Read the model definition and answer for the solid it produces. Units are mm, in the model's axes. Face numbers are marked on the shaded views. A direction names the side the tool comes from. Round coordinates to 2 decimals unless told otherwise and drop trailing zeros. Order: outer loops, then holes, each group sorted by start corner. A loop starts at its lowest first (then second) coordinate and runs counter-clockwise, first axis right, second up. Notation, with made-up numbers: (67, 37) - (81, 37) arc R26 ccw to (81, 53) - close; hole circle Ø11 at (-14, -2). An arc over 180 degrees is marked (long way). Put each result on its own line as item: value. Start each with the question number.
Q1. Section A-A on x = 103 is taken. Give the vertices of the cut face in (y, z), then the cut area to 3 significant figures.
Q2. Find the intervals of material crossed by line 1 along X through (y, z) = (216, -268); line 2 along X through (y, z) = (22, -107.5); line 3 along Z through (x, y) = (-50.5, 80.5), in increasing order. Write a range as from..to.
Q3. Which of the six approach directions +Z, -Z, +X, -X, +Y, -Y give full straight-line access (tool end or side, diameter ignored) to the marked faces 1, 2 and 3?
Q4. Section B-B on z = -290 is taken. Give the vertices of the cut face in (x, y), then the cut area to 3 significant figures.
Q5. Each of these flat-tipped pins is pushed along its axis until it touches: pin 1 Ø5.5 at (y, z) = (24.5, -353) entering from +X; pin 2 Ø5 at (x, y) = (9, -41) entering from +Z; pin 3 Ø10.5 at (x, z) = (3.5, -203.5) entering from +Y. Where does it stop, or does it pass through?
Q6. For a pull along Y with two mould halves and no side action, classify the marked faces 4, 5, 6 and 7 as pulls with the +Y half, pulls with the -Y half, needs draft (parallel to the pull), parting line crosses it, or undercut.
from build123d import *

# Parameters (mm, degrees)
SKETCH3_R           = 8.765690973
SKETCH3_R_2         = 7.546329472
BOSS_EXTRUDE1_DEPTH = 33.02
SKETCH3_3_R         = 8.765690973
SKETCH3_3_R_2       = 4.747089374
BOSS_EXTRUDE2_DEPTH = 69.85
BOSS_EXTRUDE3_START = 58.42
SKETCH3_4_R         = 8.765690973
BOSS_EXTRUDE3_DEPTH = 25.4
BOSS_EXTRUDE4_START = 147.32
SKETCH3_5_R         = 37.933984784
BOSS_EXTRUDE4_DEPTH = 88.9
BOSS_EXTRUDE5_START = -33.02
SKETCH3_6_R         = 8.765690973
BOSS_EXTRUDE5_DEPTH = 36.83
SKETCH4_R           = 29.883477217
SKETCH4_R_2         = 43.238390789
BOSS_EXTRUDE6_DEPTH = 63.5
SKETCH5_R           = 12.7
BOSS_EXTRUDE7_DEPTH = 76.2


with BuildPart() as part:
    # Sketch3 → Boss-Extrude1 (new, symmetric)
    with BuildSketch(Plane(origin=(0, 0, 0), x_dir=(0, 0, -1), z_dir=(1, 0, 0))):
        with BuildLine():
            Line((26.855598623, 34.04153134), (4.47810231, 12.180709193))
            ThreePointArc((4.47810231, 12.180709193), (-0.623125102, -0.971268934), (5.942795811, -13.456689726))
            Line((5.942795811, -13.456689726), (66.019432644, -60.042158643))
            ThreePointArc((66.019432644, -60.042158643), (76.890934177, -67.24165573), (88.712417559, -72.743912948))
            Line((88.712417559, -72.743912948), (111.45096516, -102.748262935))
            Line((111.45096516, -102.748262935), (144.477083252, -102.748262935))
            Line((144.477083252, -102.748262935), (169.002654574, -78.222691613))
            Line((169.002654574, -78.222691613), (195.607463956, -67.881296304))
            Line((195.607463956, -67.881296304), (230.151439421, -67.881296304))
            Line((230.151439421, -67.881296304), (255.413307952, -58.06190745))
            Line((255.413307952, -58.06190745), (278.88283078, -45.976265865))
            ThreePointArc((278.88283078, -45.976265865), (294.32962444, -40.865539072), (306.21453812, -29.753753007))
            Line((306.21453812, -29.753753007), (343.20837466, -16.328313428))
            Line((343.20837466, -16.328313428), (371.754392863, 12.180709193))
            Line((371.754392863, 12.180709193), (374.485546232, 37.116975937))
            Line((374.485546232, 37.116975937), (357.663762198, 55.324665065))
            Line((357.663762198, 55.324665065), (334.531136252, 76.90543329))
            Line((334.531136252, 76.90543329), (344.934785387, 122.683933603))
            Line((344.934785387, 122.683933603), (364.263564291, 181.676846378))
            Line((364.263564291, 181.676846378), (364.263564291, 198.452389962))
            Line((364.263564291, 198.452389962), (357.663762198, 223.699422208))
            Line((357.663762198, 223.699422208), (344.934785387, 227.677887566))
            Line((344.934785387, 227.677887566), (344.934785387, 233.598698071))
            Line((344.934785387, 233.598698071), (249.548191735, 247.947506817))
            Line((249.548191735, 247.947506817), (244.248903474, 242.648218557))
            Line((244.248903474, 242.648218557), (232.751756038, 242.648218557))
            Line((232.751756038, 242.648218557), (227.094867147, 224.549177586))
            Line((227.094867147, 224.549177586), (219.151380314, 218.377908492))
            Line((219.151380314, 218.377908492), (211.768889899, 192.707825641))
            Line((211.768889899, 192.707825641), (198.41781103, 192.707825641))
            Line((198.41781103, 192.707825641), (186.570468216, 151.512747216))
            Line((186.570468216, 151.512747216), (220.727605993, 147.448698974))
            Line((220.727605993, 147.448698974), (210.286236359, 90.83239142))
            Line((210.286236359, 90.83239142), (139.553233817, 50.621163948))
            Line((139.553233817, 50.621163948), (99.972286673, 57.295598172))
            Line((99.972286673, 57.295598172), (49.830851017, 45.21297855))
            Line((49.830851017, 45.21297855), (26.855598623, 34.04153134))
        make_face()
        with Locations((354.042271494, 27.57532186)):
            Circle(SKETCH3_R, mode=Mode.SUBTRACT)
        with Locations((16.377571024, 0)):
            Circle(SKETCH3_R_2, mode=Mode.SUBTRACT)
    extrude(amount=BOSS_EXTRUDE1_DEPTH, both=True)



with BuildPart() as body_2:
    # Sketch3<3> → Boss-Extrude2 (new, symmetric)
    with BuildSketch(Plane(origin=(0, 0, 0), x_dir=(0, 0, -1), z_dir=(1, 0, 0))):
        with Locations((354.042271494, 27.57532186)):
            Circle(SKETCH3_3_R)
        with Locations((354.042271494, 27.57532186)):
            Circle(SKETCH3_3_R_2, mode=Mode.SUBTRACT)
    extrude(amount=BOSS_EXTRUDE2_DEPTH, both=True)


with BuildPart() as part_1:
    add(part.part)

    add(body_2.part)  # Boss-Extrude3 merges body 2
    # Sketch3<4> → Boss-Extrude3 (add)
    with BuildSketch(Plane(origin=(0, 0, 0), x_dir=(0, 0, -1), z_dir=(1, 0, 0)).offset(BOSS_EXTRUDE3_START)):
        with BuildLine():
            ThreePointArc((32.215659867, 6.254756105), (33.341085724, 1.485328635), (33.061654594, -3.407108386))
            ThreePointArc((33.061654594, -3.407108386), (51.413629646, -45.679009257), (88.712417559, -72.743912948))
            Line((88.712417559, -72.743912948), (111.45096516, -102.748262935))
            Line((111.45096516, -102.748262935), (144.477083252, -102.748262935))
            Line((144.477083252, -102.748262935), (169.002654574, -78.222691613))
            Line((169.002654574, -78.222691613), (195.607463956, -67.881296304))
            Line((195.607463956, -67.881296304), (230.151439421, -67.881296304))
            Line((230.151439421, -67.881296304), (255.413307952, -58.06190745))
            Line((255.413307952, -58.06190745), (278.88283078, -45.976265865))
            ThreePointArc((278.88283078, -45.976265865), (294.32962444, -40.865539072), (306.21453812, -29.753753007))
            Line((306.21453812, -29.753753007), (343.20837466, -16.328313428))
            Line((343.20837466, -16.328313428), (371.754392863, 12.180709193))
            Line((371.754392863, 12.180709193), (374.485546232, 37.116975937))
            Line((374.485546232, 37.116975937), (357.663762198, 55.324665065))
            Line((357.663762198, 55.324665065), (334.531136252, 76.90543329))
            Line((334.531136252, 76.90543329), (344.934785387, 122.683933603))
            Line((344.934785387, 122.683933603), (364.263564291, 181.676846378))
            Line((364.263564291, 181.676846378), (364.263564291, 198.452389962))
            Line((364.263564291, 198.452389962), (357.663762198, 223.699422208))
            Line((357.663762198, 223.699422208), (344.934785387, 227.677887566))
            Line((344.934785387, 227.677887566), (344.934785387, 233.598698071))
            Line((344.934785387, 233.598698071), (249.548191735, 247.947506817))
            Line((249.548191735, 247.947506817), (244.248903474, 242.648218557))
            Line((244.248903474, 242.648218557), (232.751756038, 242.648218557))
            Line((232.751756038, 242.648218557), (227.094867147, 224.549177586))
            Line((227.094867147, 224.549177586), (219.151380314, 218.377908492))
            Line((219.151380314, 218.377908492), (211.768889899, 192.707825641))
            Line((211.768889899, 192.707825641), (198.41781103, 192.707825641))
            Line((198.41781103, 192.707825641), (186.570468216, 151.512747216))
            Line((186.570468216, 151.512747216), (220.727605993, 147.448698974))
            Line((220.727605993, 147.448698974), (210.286236359, 90.83239142))
            Line((210.286236359, 90.83239142), (139.553233817, 50.621163948))
            Line((139.553233817, 50.621163948), (99.972286673, 57.295598172))
            Line((99.972286673, 57.295598172), (49.830851017, 45.21297855))
            Line((49.830851017, 45.21297855), (37.556768138, 39.2448496))
            ThreePointArc((37.556768138, 39.2448496), (33.294973494, 23.007425276), (32.215659867, 6.254756105))
        make_face()
        with Locations((354.042271494, 27.57532186)):
            Circle(SKETCH3_4_R, mode=Mode.SUBTRACT)
    extrude(amount=-BOSS_EXTRUDE3_DEPTH)

    # Sketch3<5> → Boss-Extrude4 (add)
    with BuildSketch(Plane(origin=(0, 0, 0), x_dir=(0, 0, -1), z_dir=(1, 0, 0)).offset(BOSS_EXTRUDE4_START)):
        with BuildLine():
            ThreePointArc((82.075918233, 87.994388044), (19.03494718, 89.912772519), (34.422828639, 28.74858909))
            ThreePointArc((34.422828639, 28.74858909), (32.589179891, 17.57330891), (32.215659867, 6.254756105))
            ThreePointArc((32.215659867, 6.254756105), (33.341085724, 1.485328635), (33.061654594, -3.407108386))
            ThreePointArc((33.061654594, -3.407108386), (196.622426511, -32.27419595), (82.075918233, 87.994388044))
        make_face()
        with Locations(Location((274.967874889, -8.24484233, 0), (0, 0, 275.923726861))):
            Circle(SKETCH3_5_R)
    extrude(amount=-BOSS_EXTRUDE4_DEPTH)

    # Sketch3<6> → Boss-Extrude5 (add)
    with BuildSketch(Plane(origin=(0, 0, 0), x_dir=(0, 0, -1), z_dir=(1, 0, 0)).offset(BOSS_EXTRUDE5_START)):
        with BuildLine():
            ThreePointArc((32.215659867, 6.254756105), (33.341085724, 1.485328635), (33.061654594, -3.407108386))
            ThreePointArc((33.061654594, -3.407108386), (51.413629646, -45.679009257), (88.712417559, -72.743912948))
            Line((88.712417559, -72.743912948), (111.45096516, -102.748262935))
            Line((111.45096516, -102.748262935), (144.477083252, -102.748262935))
            Line((144.477083252, -102.748262935), (169.002654574, -78.222691613))
            Line((169.002654574, -78.222691613), (195.607463956, -67.881296304))
            Line((195.607463956, -67.881296304), (230.151439421, -67.881296304))
            Line((230.151439421, -67.881296304), (255.413307952, -58.06190745))
            Line((255.413307952, -58.06190745), (278.88283078, -45.976265865))
            ThreePointArc((278.88283078, -45.976265865), (294.32962444, -40.865539072), (306.21453812, -29.753753007))
            Line((306.21453812, -29.753753007), (343.20837466, -16.328313428))
            Line((343.20837466, -16.328313428), (371.754392863, 12.180709193))
            Line((371.754392863, 12.180709193), (374.485546232, 37.116975937))
            Line((374.485546232, 37.116975937), (357.663762198, 55.324665065))
            Line((357.663762198, 55.324665065), (334.531136252, 76.90543329))
            Line((334.531136252, 76.90543329), (344.934785387, 122.683933603))
            Line((344.934785387, 122.683933603), (364.263564291, 181.676846378))
            Line((364.263564291, 181.676846378), (364.263564291, 198.452389962))
            Line((364.263564291, 198.452389962), (357.663762198, 223.699422208))
            Line((357.663762198, 223.699422208), (344.934785387, 227.677887566))
            Line((344.934785387, 227.677887566), (344.934785387, 233.598698071))
            Line((344.934785387, 233.598698071), (249.548191735, 247.947506817))
            Line((249.548191735, 247.947506817), (244.248903474, 242.648218557))
            Line((244.248903474, 242.648218557), (232.751756038, 242.648218557))
            Line((232.751756038, 242.648218557), (227.094867147, 224.549177586))
            Line((227.094867147, 224.549177586), (219.151380314, 218.377908492))
            Line((219.151380314, 218.377908492), (211.768889899, 192.707825641))
            Line((211.768889899, 192.707825641), (198.41781103, 192.707825641))
            Line((198.41781103, 192.707825641), (186.570468216, 151.512747216))
            Line((186.570468216, 151.512747216), (220.727605993, 147.448698974))
            Line((220.727605993, 147.448698974), (210.286236359, 90.83239142))
            Line((210.286236359, 90.83239142), (139.553233817, 50.621163948))
            Line((139.553233817, 50.621163948), (99.972286673, 57.295598172))
            Line((99.972286673, 57.295598172), (49.830851017, 45.21297855))
            Line((49.830851017, 45.21297855), (37.556768138, 39.2448496))
            ThreePointArc((37.556768138, 39.2448496), (33.294973494, 23.007425276), (32.215659867, 6.254756105))
        make_face()
        with Locations((354.042271494, 27.57532186)):
            Circle(SKETCH3_6_R, mode=Mode.SUBTRACT)
    extrude(amount=-BOSS_EXTRUDE5_DEPTH)

    # Sketch4 → Boss-Extrude6 (add)
    with BuildSketch(Plane.ZY.offset(69.85)):
        with Locations(Location((-167.668024488, 31.122707437, 0), (0, 0, 180))):
            Circle(SKETCH4_R)
        with Locations(Location((-226.332433107, -21.383558841, 0), (0, 0, 180))):
            Circle(SKETCH4_R_2)
    extrude(amount=BOSS_EXTRUDE6_DEPTH)

    # Sketch5 → Boss-Extrude7 (add)
    with BuildSketch(Plane(origin=(0, 279.169325886, -41.994866484), x_dir=(1, 0, 0), z_dir=(0, 0.9888741863075109, -0.1487543063398786))):
        with Locations(Location((0, 269.608209436, 0), (0, 0, 270))):
            Circle(SKETCH5_R)
    extrude(amount=BOSS_EXTRUDE7_DEPTH)


solid = part_1.part
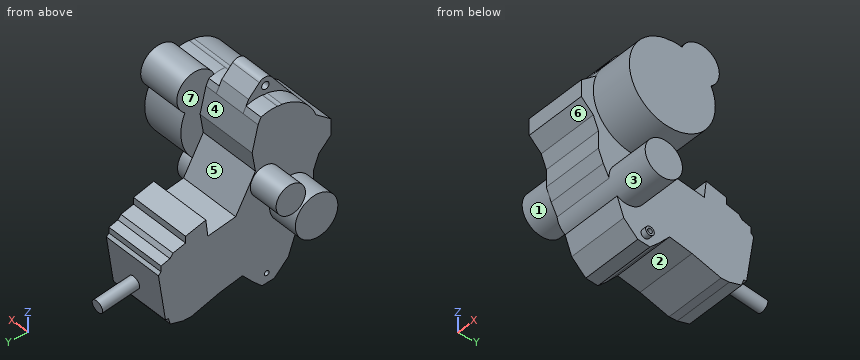
Findings:
1. outline: circle Ø75.87 at (-8.24, -274.97); (-3.41, -33.06) arc R87.41 ccw (long way) to (87.99, -82.08) arc R39.52 ccw (long way) to (28.75, -34.42) arc R87.41 ccw to (6.25, -32.22) arc R17.03 cw to start
1. area: 31,400 mm2
2. line 1: -69.85..58.42
2. line 2: -69.85..147.32
2. line 3: -335.35..-192.11
3. face 1: -X
3. face 2: -Z, +X, -X
3. face 3: +X
4. outline: (-69.85, -43.07) - (147.32, -43.07) - (147.32, 26.58) - (58.42, 26.58) - (58.42, 241.86) - (-69.85, 241.86) - close
4. area: 42,700 mm2
5. pin 1: x = 69.85
5. pin 2: z = -38.24
5. pin 3: y = 192.71
6. face 4: pulls with the +Y half
6. face 5: undercut
6. face 6: pulls with the -Y half
6. face 7: needs draft
